Answer from the drawing. Dimensions are ordinates in mm from the lowest x, y and z of the part. A direction names the side the tool comes from. Coordinates: 2 decimals unless noted, no trailing zeros. Order: outer loops, then holes, each group sorted by start corner. A loop starts at its lowest first (then second) coordinate and runs counter-clockwise, first axis right, second up.
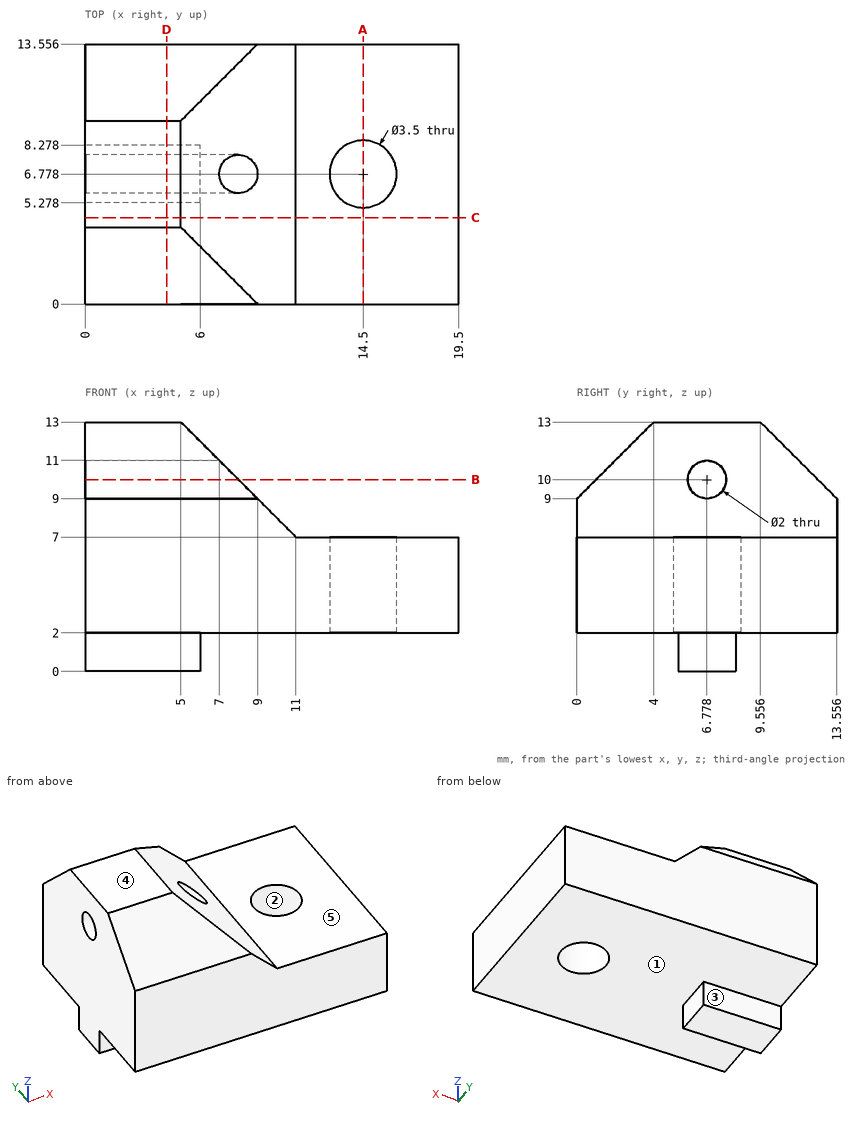
1) Section B-B (z = 10) is taken. Give the vertices of the cut face in (x, y).
2) A tool of negligible diameter and unlimited length cuts with its end or side. For the marked faces 4 and 5, from which of +Z, -Z, +X, -X, +Y, -Y can it reach the whole face along a straight path? Write none if from no direction.
3) Consider L1, parallel to Y at x = 14.5, z = 5.1; L2, parallel to Z at x = 17, y = 0.75; L3, parallel to Z at x = 2, y = 7.25. Determine where each line is inside the solid, lowest interval first.
4) Determine the mould class of the marked faces 1, 2 and 3 for opening direction Y: released by +Y, released by -Y, zero draft, split by the parting line, or undercut.
5) Section A-A (x = 14.5) is taken. Give the vertices of the cut face in (y, z), then the cut area to 3 significant figures.
6) Section C-C (y = 4.5) is taken. Give the vertices of the cut face in (x, z), then the cut area to 4 significant figures.
7) Section D-D (x = 4.25) is taken. Give the vertices of the cut face in (y, z).
8) Each of these flat-tipped pins is pushed along its axis until it touches: P1, Ø5, axis at x = 15.5, y = 10, coming from the -Z side; P2, Ø1, axis at x = 2.5, z = 1, coming from the +Y side; P3, Ø1, axis at y = 2.5, z = 9.5, coming from the +X side. Where does it stop, or does it pass through?
Filled sheet:
1. outline: (0, 1) - (8, 1) - (8, 5.78) - (0, 5.78) - close; (0, 7.78) - (8, 7.78) - (8, 12.56) - (0, 12.56) - close
2. face 4: +Z, +X, -X, +Y, -Y
2. face 5: +Z, +X, +Y, -Y
3. L1: y = 0 to 5.03, 8.53 to 13.56
3. L2: z = 2 to 7
3. L3: z = 0 to 9.12, 10.88 to 13
4. face 1: zero draft
4. face 2: undercut
4. face 3: released by +Y
5. outline: (0, 2) - (5.03, 2) - (5.03, 7) - (0, 7) - close; (8.53, 2) - (13.56, 2) - (13.56, 7) - (8.53, 7) - close
5. area: 50.3 mm2
6. outline: (0, 2) - (19.5, 2) - (19.5, 7) - (11, 7) - (5, 13) - (0, 13) - close
6. area: 145.5 mm2
7. outline: (0, 2) - (5.28, 2) - (5.28, 0) - (8.28, 0) - (8.28, 2) - (13.56, 2) - (13.56, 9) - (9.56, 13) - (4, 13) - (0, 9) - close; hole circle Ø2 at (6.78, 10)
8. P1: stops at z = 2
8. P2: stops at y = 8.28
8. P3: stops at x = 9
